```python
from build123d import *

# Parameters (mm, degrees)
SKETCH1_R           = 2
BOSS_EXTRUDE1_DEPTH = 16
SKETCH2_R           = 3.2
BOSS_EXTRUDE2_DEPTH = 1.7
BOSS_EXTRUDE2_TAPER = 32
SKETCH3_W           = 0.5
SKETCH3_H           = 2.258378485
SKETCH3_H_2         = 2.241621515
SKETCH3_W_2         = 2.234727157
SKETCH3_H_3         = 0.5
SKETCH3_W_3         = 2.265272843
CUT_EXTRUDE1_DEPTH  = 0.3


with BuildPart() as part:
    # Sketch1 → Boss-Extrude1 (new body)
    with BuildSketch(Plane(origin=(0, 0, 0), x_dir=(1, 0, 0), z_dir=(0, 1, 0))):
        Circle(SKETCH1_R)
    extrude(amount=BOSS_EXTRUDE1_DEPTH)

    # Sketch2 → Boss-Extrude2 (add)
    with BuildSketch(Plane(origin=(0, 16, 0), x_dir=(1, 0, 0), z_dir=(0, 1, 0))):
        Circle(SKETCH2_R)
    extrude(amount=-BOSS_EXTRUDE2_DEPTH, taper=BOSS_EXTRUDE2_TAPER)

    # Sketch3 → Cut-Extrude1 (cut)
    with BuildSketch(Plane(origin=(0, 16, 0), x_dir=(1, 0, 0), z_dir=(0, 1, 0))):
        with Locations((-0.015272843, 1.370810757)):
            Rectangle(SKETCH3_W, SKETCH3_H)
        with Locations((-0.015272843, -1.379189243)):
            Rectangle(SKETCH3_W, SKETCH3_H_2)
        with Locations((-1.382636421, -0.008378485)):
            Rectangle(SKETCH3_W_2, SKETCH3_H_3)
        with Locations((1.367363579, -0.008378485)):
            Rectangle(SKETCH3_W_3, SKETCH3_H_3)
        with Locations((-0.015272843, -0.008378485)):
            Rectangle(SKETCH3_W, SKETCH3_H_3)
    extrude(amount=-CUT_EXTRUDE1_DEPTH, mode=Mode.SUBTRACT)


solid = part.part
```
CAD build for the part. Positions are in the model's coordinates, mm. A direction names the side the tool comes from. Give positions to 0.01 mm unless a question says otherwise; leave off trailing zeros. Write each loop counter-clockwise with the first axis right and the second up, starting at its lowest first coordinate (ties: lowest second). Pieces come first, ordered by that corner, then holes. Notation, with made-up numbers: M 59,9.25 L 95,9.25 A31 ccw 95,38.25 Z; hole C 34.5,-38 d2. An arc over 180 degrees is marked long. Return JSON: item names as keys, results as strings. Group by question number.
(1) 3-axis set-ups, long thin cutter, end or side, ignore diameter. For faces 1 (the face through (0, 0, 0)), 2 (the face through (0, 7, 2)): which of +Z, -Z, +X, -X, +Y, -Y reach the whole face in a straight line?
(2) Band-saw the part on A-A (x = 0). Give the cut face in (y, z).
(3) Drill centre lines: L1, parallel to Y at x = -1, z = 0; L2, parallel to X at y = 6.75, z = 0; L3, parallel to Z at x = -0.25, y = 11.75. Where is each one in solid material? Low to high. Write a range as [from, to].
(4) Band-saw the part on B-B (y = 12.75). Give the cut face in (x, z).
(5) Flat gauge pins, fed straight in: pin 1 Ø2 at (x, z) = (-2.5, -2.5) entering from -Y; pin 2 Ø2 at (x, z) = (0, -0.5) entering from -Y; pin 3 Ø2 at (x, y) = (-1, 3.5) entering from -Z; pin 4 Ø2 at (y, z) = (8.5, 2) entering from +X. Where does each tip first touch, or does it go through?
(6) Band-saw the part on C-C (y = 15). Give the cut face in (x, z), and give its area (3 significant figures).
Entries:
{
 "1": {"face 1": "+Z, -Z, +X, -X, -Y", "face 2": "-Y"},
 "2": {"outline": "M 0,-2 L 14.3,-2 L 14.3,-2.14 L 16,-3.2 L 16,-2.5 L 15.7,-2.5 L 15.7,2.5 L 16,2.5 L 16,3.2 L 14.3,2.14 L 14.3,2 L 0,2 Z"},
 "3": {"L1": "y = [0, 15.7]", "L2": "x = [-2, 2]", "L3": "z = [-1.98, 1.98]"},
 "4": {"outline": "C 0,0 d4"},
 "5": {"pin 1": "stops at y = 14.94", "pin 2": "stops at y = 0", "pin 3": "stops at z = -2", "pin 4": "stops at x = 1.73"},
 "6": {"outline": "C 0,0 d5.15", "area": "20.8 mm^2"}
}
